Verification items for the finished model (mm, model axes). A direction names the side the tool comes from. Coordinates: 2 decimals unless noted, no trailing zeros. Loops run counter-clockwise (first coordinate to the right, second up) from the corner with the lowest first, then second, coordinate; pieces in that order, holes last. Notation, with made-up numbers: (26, 74.25) -> (66, 74.25) arc R19 ccw to (66, 95.25) -> close; hole circle Ø2 at (-24.5, 82.5). An arc over 180 degrees is marked (long way). Answer as a JSON object with one key per item and string values. Group by question number.
Q1. Cross-section at C-C on y = 170. Record the boundary of the cut face in (x, z).
Q2. Cross-section at A-A on x = -83.5. Record the boundary of the cut face in (y, z).
Q3. Scan lines: L1, parallel to Z at x = -80, y = 158.5; L2, parallel to Y at x = -149, z = 73.5. Record each from-to range of solid material in increasing order.
Q4. Set-up check for faces 1 (the flat face through (-113, 182.033, 104)), 2 (the flat face through (-113, 181, 0)): record each of +Z, -Z, +X, -X, +Y, -Y from which the full face is reachable in a straight line by a thin tool's end or side.
Q5. Gauge pin test, flat ends, axial feed: pin 1 Ø6 at (x, z) = (-28, 114) entering from -Y; pin 2 Ø10 at (x, y) = (-198, 109.5) entering from +Z. Record the tip position at first contact, or that the pin passes through.
Q6. Cross-section at B-B on z = 128. Record the boundary of the cut face in (x, y), and give its area (3 significant figures).
```python
from build123d import *

# Parameters (mm, degrees)
F0_W     = 273.05
F0_H     = 228.6
F1_DEPTH = 228.6
F3_DEPTH = 228.6


with BuildPart() as f1:
    # F0 (on Right) → F1 (new body)
    with BuildSketch(Plane.YZ):
        with Locations((136.525, 114.3)):
            Rectangle(F0_W, F0_H)
    extrude(amount=-F1_DEPTH)

    # F2 (on face) → F3 (cut, through all)
    with BuildSketch(Plane.YZ):
        Polygon((182.033333, 139.7), (273.05, 139.7), (273.05, 228.6), (0, 228.6), (0, 0), (91.016667, 0), (91.016667, 69.85), (182.033333, 69.85), align=None)
    extrude(amount=-F3_DEPTH, mode=Mode.SUBTRACT)


solid = f1.part
```
Computed values:
{
 "1": {"outline": "(-228.6, 0) -> (0, 0) -> (0, 69.85) -> (-228.6, 69.85) -> close"},
 "2": {"outline": "(91.02, 0) -> (273.05, 0) -> (273.05, 139.7) -> (182.03, 139.7) -> (182.03, 69.85) -> (91.02, 69.85) -> close"},
 "3": {"L1": "z = 0 to 69.85", "L2": "y = 182.03 to 273.05"},
 "4": {"face 1": "+Z, +X, -X, -Y", "face 2": "-Z, +X, -X, +Y, -Y"},
 "5": {"pin 1": "stops at y = 182.03", "pin 2": "stops at z = 69.85"},
 "6": {"outline": "(-228.6, 182.03) -> (0, 182.03) -> (0, 273.05) -> (-228.6, 273.05) -> close", "area": "20,800 mm²"}
}
